Verification items for the finished model (mm, model axes). Face numbers are marked on the shaded views. A direction names the side the tool comes from. Coordinates: 2 decimals unless noted, no trailing zeros. Write each loop counter-clockwise with the first axis right and the second up, starting at its lowest first coordinate (ties: lowest second). Pieces come first, ordered by that corner, then holes. Notation, with made-up numbers: (50, -2.75) -> (87, -2.75) arc R29 cw to (87, 31.25) -> close; hole circle Ø4 at (20, 19.25). An arc over 180 degrees is marked (long way). Use a Markdown table: item, result. Add a question column.
from build123d import *

# Parameters (mm, degrees)
EXTRUDE_1_DEPTH          = 20
SKETCH_2_W               = 16
SKETCH_2_H               = 16
EXTRUDE_2_DEPTH          = 3
CUT_EXTRUDE_1_DEPTH      = 26.632011236
RIB_1_REACH              = 27.632
SKETCH_4_WALL_W          = 56.799556378
SKETCH_4_WALL_H          = 2
PATTERN_CIRCULAR_1_COUNT = 4
EXTRUDE_3_DEPTH          = 2
PATTERN_LINEAR_1_COUNT   = 2
PATTERN_LINEAR_1_PITCH   = 8
MIRROR_1_COPY_1_DEPTH    = 2
FILLET_1_R               = 2
FILLET_2_R               = 0.2
FILLET_4_R               = 0.2
HOLE_WIZARD_M3_1_D       = 2.5
CUT_EXTRUDE_2_DEPTH      = 27.139051364
CUT_EXTRUDE_2_DEPTH_BACK = 27.139051364
SKETCH_11_R              = 1.25
SKETCH_12_R              = 1.75
CUT_EXTRUDE_3_DEPTH      = 2
CUT_EXTRUDE_4_DEPTH      = 2
CUT_EXTRUDE_5_DEPTH      = 8


with BuildPart() as part:
    # 草图1 → 凸台-拉伸1 (new body)
    with BuildSketch(Plane(origin=(0, 0, 0), x_dir=(1, 0, 0), z_dir=(0, 1, 0))):
        with BuildLine():
            Line((-0.25, 8), (-0.25, 4.242640687))
            ThreePointArc((-0.25, 4.242640687), (0, -4.25), (0.25, 4.242640687))
            Line((0.25, 4.242640687), (0.25, 8))
            Line((0.25, 8), (1.5, 8))
            Line((1.5, 8), (1.5, 5.291502622))
            ThreePointArc((1.5, 5.291502622), (0, -5.5), (-1.5, 5.291502622))
            Line((-1.5, 5.291502622), (-1.5, 8))
            Line((-1.5, 8), (-0.25, 8))
        make_face()
    extrude(amount=EXTRUDE_1_DEPTH)

    # 草图2 → 凸台-拉伸2 (add)
    with BuildSketch(Plane(origin=(0, 20, 0), x_dir=(1, 0, 0), z_dir=(0, 1, 0))):
        Rectangle(SKETCH_2_W, SKETCH_2_H)
    extrude(amount=EXTRUDE_2_DEPTH)

    # 草图3 → 切除-拉伸1 (cut, through all)
    with BuildSketch(Plane.XZ):
        with BuildLine():
            Line((-0.25, -8), (0.25, -8))
            Line((0.25, -8), (0.25, -4.242640687))
            ThreePointArc((0.25, -4.242640687), (0, 4.25), (-0.25, -4.242640687))
            Line((-0.25, -4.242640687), (-0.25, -8))
        make_face()
    extrude(amount=-CUT_EXTRUDE_1_DEPTH, mode=Mode.SUBTRACT)

    # 草图4 wall → 筋1 (add, up to next)
    with BuildSketch(Plane(origin=(-6.75, 18.75, 0), x_dir=(0.707106781187, -0.707106781187, 0), z_dir=(0.707106781187, 0.707106781187, 0)), mode=Mode.PRIVATE) as rib_1_sk1:
        Rectangle(SKETCH_4_WALL_W, SKETCH_4_WALL_H)
    rib_1_tool1 = extrude(rib_1_sk1.sketch, amount=RIB_1_REACH, mode=Mode.PRIVATE) - part.part
    rib_1 = rib_1_tool1.solids().sort_by_distance((-6.75, 18.75, 0))[0]
    add(rib_1)

    # 阵列(圆周)1: 筋1 ×4 about axis, 1 skipped
    pattern_circular_1_axis = Axis((0, 0, 0), (0, 1, 0))
    add([rib_1.rotate(pattern_circular_1_axis, i * 360 / PATTERN_CIRCULAR_1_COUNT) for i in range(1, PATTERN_CIRCULAR_1_COUNT) if i not in (3,)])

    # 草图6 → 凸台-拉伸3 (add)
    with BuildSketch(Plane(origin=(0, 5, 0), x_dir=(1, 0, 0), z_dir=(0, 1, 0))):
        with BuildLine():
            Line((-1.5, 8), (-4.066385849, 3.703310158))
            ThreePointArc((-4.066385849, 3.703310158), (-2.894261854, 4.676884467), (-1.5, 5.291502622))
            Line((-1.5, 5.291502622), (-1.5, 8))
        make_face()
    extrude_3 = extrude(amount=EXTRUDE_3_DEPTH)

    # 阵列(线性)1: 凸台-拉伸3 ×2
    with Locations(*[(0, i * PATTERN_LINEAR_1_PITCH, 0) for i in range(1, PATTERN_LINEAR_1_COUNT)]):
        add(extrude_3)

    # 镜向1: 凸台-拉伸3 across plane
    add(extrude_3.mirror(Plane(origin=(0, 0, 0), x_dir=(0, 0, 1), z_dir=(1, 0, 0))))

    # 镜向1 copy 1 sketch → 镜向1 copy 1 (add)
    with BuildSketch(Plane(origin=(0, 13, 0), x_dir=(-1, 0, 0), z_dir=(0, 1, 0))):
        with BuildLine():
            Line((-1.5, -8), (-4.066385849, -3.703310158))
            ThreePointArc((-4.066385849, -3.703310158), (-2.894261854, -4.676884467), (-1.5, -5.291502622))
            Line((-1.5, -5.291502622), (-1.5, -8))
        make_face()
    extrude(amount=MIRROR_1_COPY_1_DEPTH)

    # 圆角1
    fillet_1_edges = [part.edges().sort_by_distance(p)[0] for p in [
        (-8, 21.5, -8),
        (-8, 21.5, 8),
        (8, 21.5, 8),
        (8, 21.5, -8),
    ]]
    fillet(fillet_1_edges, radius=FILLET_1_R)

    # 圆角2
    fillet_2_edges = [part.edges().sort_by_distance(p)[0] for p in [
        (-0.25, 10, -8),
        (0.25, 10, -8),
    ]]
    fillet(fillet_2_edges, radius=FILLET_2_R)

    # 圆角4
    fillet_4_edges = [part.edges().sort_by_distance(p)[0] for p in [
        (3.225, 23, -8),
        (8, 23, 0),
        (-8, 23, 0),
        (0, 23, 8),
        (-7.414213562, 23, -7.414213562),
        (-7.414213562, 23, 7.414213562),
        (7.414213562, 23, 7.414213562),
        (7.414213562, 23, -7.414213562),
        (0.25, 23, -6.021320344),
        (-3.225, 23, -8),
        (-0.308578644, 23, -7.941421356),
        (0.308578644, 23, -7.941421356),
        (-0.25, 23, -6.021320344),
    ]]
    fillet(fillet_4_edges, radius=FILLET_4_R)

    # M3 螺纹孔的螺纹孔钻头1 (through all)
    with Locations(Plane(origin=(0, 20, 0), x_dir=(-1, 0, 0), z_dir=(0, -1, 0))):
        with Locations((6, 6), (6, -6), (-6, 6), (-6, -6)):
            Hole(HOLE_WIZARD_M3_1_D / 2)

    # 草图11 → 切除-拉伸2 (cut, two sides: drawn at the far end of the back side and taken through both)
    with BuildSketch(Plane.ZY.offset(1.5).offset(-CUT_EXTRUDE_2_DEPTH_BACK)):
        with Locations(Location((-6, 17.5, 0), (0, 0, 304.527234227))):
            Circle(SKETCH_11_R)
        with Locations(Location((-6, 10, 0), (0, 0, 304.527234227))):
            Circle(SKETCH_11_R)
        with Locations(Location((-6, 2.5, 0), (0, 0, 304.527234227))):
            Circle(SKETCH_11_R)
    extrude(amount=CUT_EXTRUDE_2_DEPTH + CUT_EXTRUDE_2_DEPTH_BACK, mode=Mode.SUBTRACT)

    # 草图12 → 切除-拉伸3 (cut)
    with BuildSketch(Plane.ZY.offset(1.5)):
        with Locations((-6, 17.5)):
            Circle(SKETCH_12_R)
        with Locations((-6, 10)):
            Circle(SKETCH_12_R)
        with Locations((-6, 2.5)):
            Circle(SKETCH_12_R)
    extrude(amount=CUT_EXTRUDE_3_DEPTH, mode=Mode.SUBTRACT)

    # 草图13 → 切除-拉伸4 (cut)
    with BuildSketch(Plane(origin=(1.5, 0, 0), x_dir=(0, 0, -1), z_dir=(1, 0, 0))):
        Polygon((6, 19.520725942), (4.25, 18.510362971), (4.25, 16.489637029), (6, 15.479274058), (7.75, 16.489637029), (7.75, 18.510362971), align=None)
        Polygon((6, 12.020725942), (4.25, 11.010362971), (4.25, 8.989637029), (6, 7.979274058), (7.75, 8.989637029), (7.75, 11.010362971), align=None)
        Polygon((6, 4.520725942), (4.25, 3.510362971), (4.25, 1.489637029), (6, 0.479274058), (7.75, 1.489637029), (7.75, 3.510362971), align=None)
    extrude(amount=CUT_EXTRUDE_4_DEPTH, mode=Mode.SUBTRACT)

    # 草图16 → 切除-拉伸5 (cut)
    with BuildSketch(Plane.XY.offset(8)):
        with BuildLine():
            Line((-3.8, 19), (-1.7, 19))
            ThreePointArc((-1.7, 19), (-1.558578644, 18.941421356), (-1.5, 18.8))
            Line((-1.5, 18.8), (-1.5, 17.7))
            ThreePointArc((-1.5, 17.7), (-1.558578644, 17.558578644), (-1.7, 17.5))
            Line((-1.7, 17.5), (-3.8, 17.5))
            ThreePointArc((-3.8, 17.5), (-3.941421356, 17.558578644), (-4, 17.7))
            Line((-4, 17.7), (-4, 18.8))
            ThreePointArc((-4, 18.8), (-3.941421356, 18.941421356), (-3.8, 19))
        make_face()
        with BuildLine():
            Line((1.5, 18.8), (1.5, 17.7))
            ThreePointArc((1.5, 17.7), (1.558578644, 17.558578644), (1.7, 17.5))
            Line((1.7, 17.5), (3.8, 17.5))
            ThreePointArc((3.8, 17.5), (3.941421356, 17.558578644), (4, 17.7))
            Line((4, 17.7), (4, 18.8))
            ThreePointArc((4, 18.8), (3.941421356, 18.941421356), (3.8, 19))
            Line((3.8, 19), (1.7, 19))
            ThreePointArc((1.7, 19), (1.558578644, 18.941421356), (1.5, 18.8))
        make_face()
    extrude(amount=-CUT_EXTRUDE_5_DEPTH, mode=Mode.SUBTRACT)


solid = part.part
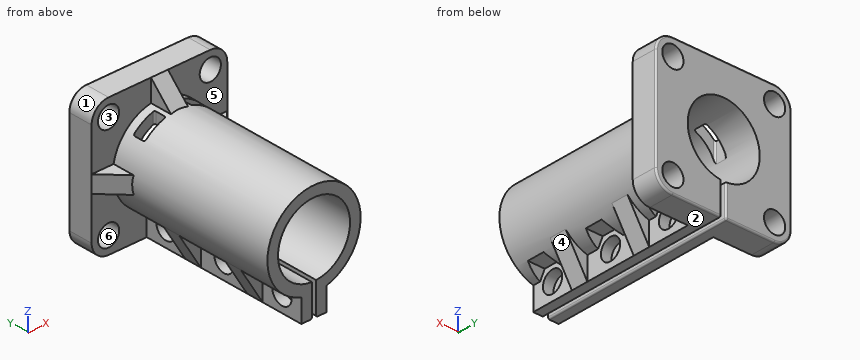
1) Cross-section at A-A on z = 0. Record the boundary of the cut face in (x, y), then the cut area to 3 significant figures.
2) Cross-section at B-B on y = 21.5. Record the boundary of the cut face in (x, z).
3) Release check for a two-part mould opening along X. For the marked faces 1, 2 and 3 record: released by +X, released by -X, zero draft, split by the parting line, or undercut.
4) Gauge pin test, flat ends, axial feed: pin 1 (3 mm diameter, centred on y = 10, z = -7, fed in from +X); pin 2 (1.5 mm diameter, centred on x = 5.5, y = 9, fed in from -Z); pin 3 (8 mm diameter, centred on x = -4.5, y = 4, fed in from +Z). Record the tip position at first contact, or that the pin passes through.
5) Cross-section at C-C on y = 2.25. Record the boundary of the cut face in (x, z).
6) Thickness scan on L1, parallel to Y at x = 1.2, z = -6; L2, parallel to X at y = 21.6, z = -6; L3, parallel to X at y = 11.75, z = 0. Record the ranges inside material, lowest first.
7) Cross-section at D-D on z = -2. Record the boundary of the cut face in (x, y), then the cut area to 3 significant figures.
8) Set-up check for the marked faces 4, 5 and 6: record each of +Z, -Z, +X, -X, +Y, -Y from which the full face is reachable in a straight line by a thin tool's end or side.
Returned:
| question | item | result |
|---|---|---|
| 1 | outline | (-8, 20) -> (-5.5, 17.5) -> (-5.5, 0) -> (-4.25, 0) -> (-4.25, 23) -> (-7.8, 23) arc R0.2 ccw to (-8, 22.8) -> close; (4.25, 0) -> (5.5, 0) -> (5.5, 17.5) -> (8, 20) -> (8, 22.8) arc R0.2 ccw to (7.8, 23) -> (4.25, 23) -> close |
| 1 | area | 78.7 mm² |
| 2 | outline | (-8, -6) arc R2 ccw to (-6, -8) -> (-0.45, -8) arc R0.2 ccw to (-0.25, -7.8) -> (-0.25, -4.24) arc R4.25 cw (long way) to (0.25, -4.24) -> (0.25, -7.8) arc R0.2 ccw to (0.45, -8) -> (6, -8) arc R2 ccw to (8, -6) -> (8, 6) arc R2 ccw to (6, 8) -> (-6, 8) arc R2 ccw to (-8, 6) -> close; hole circle Ø2.5 at (-6, -6); hole circle Ø2.5 at (-6, 6); hole circle Ø2.5 at (6, -6); hole circle Ø2.5 at (6, 6) |
| 3 | face 1 | released by -X |
| 3 | face 2 | zero draft |
| 3 | face 3 | undercut |
| 4 | pin 1 | stops at x = 1.5 |
| 4 | pin 2 | stops at z = -2.77 |
| 4 | pin 3 | stops at z = 5.48 |
| 5 | outline | (-3.47, -4.27) -> (-1.5, -4.27) -> (-1.5, -4.78) -> (-0.25, -4.78) -> (-0.25, -4.24) arc R4.25 cw (long way) to (0.25, -4.24) -> (0.25, -4.78) -> (1.5, -4.78) -> (1.5, -4.25) -> (3.49, -4.25) arc R5.5 ccw (long way) to start; (-1.5, -8) -> (-0.45, -8) arc R0.2 ccw to (-0.25, -7.8) -> (-0.25, -7.22) -> (-1.5, -7.22) -> close; (0.25, -7.8) arc R0.2 ccw to (0.45, -8) -> (1.5, -8) -> (1.5, -7.22) -> (0.25, -7.22) -> close |
| 6 | L1 | y = 0 to 1.25, 3.75 to 8.75, 11.25 to 16.25, 18.75 to 23 |
| 6 | L2 | x = -8 to -7.25, -4.75 to -0.25, 0.25 to 4.75, 7.25 to 8 |
| 6 | L3 | x = -5.5 to -4.25, 4.25 to 5.5 |
| 7 | outline | (-8, 20) -> (-5.12, 20) -> (-5.12, 0) -> (-3.75, 0) -> (-3.75, 23) -> (-7.8, 23) arc R0.2 ccw to (-8, 22.8) -> close; (3.75, 0) -> (5.12, 0) -> (5.12, 20) -> (8, 20) -> (8, 22.8) arc R0.2 ccw to (7.8, 23) -> (3.75, 23) -> close |
| 7 | area | 80.4 mm² |
| 8 | face 4 | -Z, +X, -Y |
| 8 | face 5 | +Z, +X, -Y |
| 8 | face 6 | +Y, -Y |
